```python
from build123d import *

# Parameters (mm, degrees)
F2_R      = 17.5
F3_DEPTH  = 28
F4_T      = -2
F6_D      = 3.3
F2_R_2    = 34
F7_DEPTH  = 2
F9_D      = 2.5
F10_DEPTH = 2


with BuildPart() as f3:
    # F2 (on Top) → F3 (new body)
    with BuildSketch(Plane.XY):
        Circle(F2_R)
    extrude(amount=F3_DEPTH)

    # F4
    f4_openings = [f3.faces().sort_by_distance(p)[0] for p in [
        (0, 0, 0),
    ]]
    offset(amount=F4_T, openings=f4_openings)

    # F6 (through all)
    with Locations(Plane.XY.offset(28)):
        with Locations((0, 8), (-9.5, 0), (0, -8), (9.5, 0)):
            Hole(F6_D / 2)

    # F2 (on Top) → F7 (join)
    with BuildSketch(Plane.XY):
        Circle(F2_R_2)
        Circle(F2_R, mode=Mode.SUBTRACT)
    extrude(amount=F7_DEPTH)

    # F9 (through all)
    with Locations(Plane.XY.offset(2)):
        with Locations((-6.2225225174, 30.3406529148), (-27.6628416756, 13.9299029504), (-28.0808143116, -13.0668616498), (-7.1588025741, -30.1334789143), (19.2035334136, -24.3001915673), (30.972165016, 0), (3.7694229457, 30.7419331928)):
            Hole(F9_D / 2)

    # F5 (on face) → F10 (cut, through all)
    with BuildSketch(Plane.XY.offset(28)):
        with BuildLine():
            ThreePointArc((2.4031919002, -2.5445370288), (2.6811555509, 2.2497566339), (-2.0885698997, 2.8085362333))
            Line((-2.0885698997, 2.8085362333), (-15.8475312913, -7.4233248596))
            ThreePointArc((-15.8475312913, -7.4233248596), (-13.4057777546, -11.2487831695), (-10.0624428041, -14.3177248477))
            Line((-10.0624428041, -14.3177248477), (2.4031919002, -2.5445370288))
        make_face()
    extrude(amount=-F10_DEPTH, mode=Mode.SUBTRACT)


solid = f3.part
```
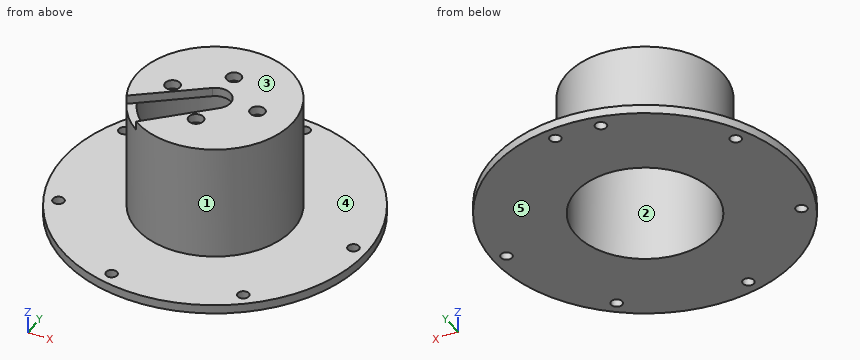
Source: CAD feature listing. Evaluate the final solid. Frame: model axes, mm. Face numbers are marked on the shaded views. A direction names the side the tool comes from. Round coordinates to 2 decimals unless told otherwise and drop trailing zeros. Loops run counter-clockwise (first coordinate to the right, second up) from the corner with the lowest first, then second, coordinate; pieces in that order, holes last.
1. Section query A-A on y = 8. Output: boundary loops of the cut face in (x, z), and give its area (3 significant figures).
2. Section query B-B on x = 9.5. Output: boundary loops of the cut face in (y, z), and give its area (3 significant figures).
3. Mould query, pull axis Y, two halves, no side actions, for the marked faces 1, 2 and 3. Classes: released by +Y, released by -Y, zero draft, split by the parting line, or undercut.
4. Section query C-C on y = 0. Output: boundary loops of the cut face in (x, z), and give its area (3 significant figures).
5. Section query D-D on z = 6.5. Output: boundary loops of the cut face in (x, y), and give its area (3 significant figures).
6. Access query for the marked faces 4 and 5. Directions: +Z, -Z, +X, -X, +Y, -Y. A direction counts if a zero-diameter tool reaches every point of the face in a straight line with its end or side. Return the directions, or none.
7. Contact query for flat-ended pins moving along their axis: pin 1 (12 mm diameter, centred on x = -2, z = 13, fed in from -Y); pin 2 (3 mm diameter, centred on x = -28.08, y = -13.07, fed in from +Z); pin 3 (6 mm diameter, centred on x = 17, z = 18, fed in from -Y). Output: stop coordinate, or through.
8. Ray query, L1, parallel to Y at x = 0, z = 27.3; L2, parallel to X at y = 0, z = 17; L3, parallel to Z at x = 4, y = -22.5. Return the intervals inside material, ascending.
Answers below:
1. outline: (-33.05, 0) - (-13.28, 0) - (-13.28, 26) - (-1.65, 26) - (-1.65, 28) - (-15.56, 28) - (-15.56, 2) - (-33.05, 2) - close; (1.65, 26) - (13.28, 26) - (13.28, 0) - (33.05, 0) - (33.05, 2) - (15.56, 2) - (15.56, 28) - (1.65, 28) - close
1. area: 245 mm2
2. outline: (-32.65, 0) - (-12.25, 0) - (-12.25, 26) - (-1.65, 26) - (-1.65, 28) - (-14.7, 28) - (-14.7, 2) - (-32.65, 2) - close; (1.65, 26) - (12.25, 26) - (12.25, 0) - (32.65, 0) - (32.65, 2) - (14.7, 2) - (14.7, 28) - (1.65, 28) - close
2. area: 251 mm2
3. face 1: split by the parting line
3. face 2: undercut
3. face 3: zero draft
4. outline: (-34, 0) - (-15.5, 0) - (-15.5, 26) - (-11.15, 26) - (-11.15, 28) - (-17.5, 28) - (-17.5, 2) - (-34, 2) - close; (-7.85, 26) - (-5.87, 26) - (-5.87, 28) - (-7.85, 28) - close; (3.5, 26) - (7.85, 26) - (7.85, 28) - (3.5, 28) - close; (11.15, 26) - (15.5, 26) - (15.5, 0) - (29.72, 0) - (29.72, 2) - (17.5, 2) - (17.5, 28) - (11.15, 28) - close; (32.22, 0) - (34, 0) - (34, 2) - (32.22, 2) - close
4. area: 203 mm2
5. outline: circle Ø35 at (0, 0); hole circle Ø31 at (0, 0)
5. area: 207 mm2
6. face 4: +Z
6. face 5: -Z, +X, -X, +Y, -Y
7. pin 1: stops at y = -17.5
7. pin 2: stops at z = 2
7. pin 3: stops at y = -10.5
8. L1: y = -17.5 to -9.65, -6.35 to -4.81, 3.5 to 6.35, 9.65 to 17.5
8. L2: x = -17.5 to -15.5, 15.5 to 17.5
8. L3: z = 0 to 2
